Autodesk Inventor part; units mm, degrees
ref_plane "YZ Plane" through (0, 0, 0) normal (1, 0, 0) x (0, 1, 0)
ref_plane "XZ Plane" through (0, 0, 0) normal (0, 1, 0) x (-1, 0, 0)
ref_plane "XY Plane" through (0, 0, 0) normal (0, 0, 1) x (1, 0, 0)
ref_plane "Work Plane1" through (0, 0, 2) normal (0, 0, 1) x (1, 0, 0)
sketch "Sketch1" plane through (0, 0, 2) normal (0, 0, 1) x (1, 0, 0)
  circle A0 centre (-37.0712, 14) radius 3.25 construction
  circle A1 centre (-9.0712, -14) radius 3.25 construction
  line L0 (-21.8762, -24.9) -> (-21.8762, -17.08) construction
  line L1 (-21.8762, -17.08) -> (-20.0712, -17.08) construction
  arc A2 (-20.0712, -17.08) -> (-20.0712, -14.08) centre (-20.0712, -15.58) ccw construction
  line L2 (-20.0712, -14.08) -> (-21.8762, -14.08) construction
  line L3 (-21.8762, -14.08) -> (-21.8762, -3.0223) construction
  arc A3 (-21.8762, -3.0223) -> (-25.9925, 1.4242) centre (-23.0712, 0) ccw construction
  line L4 (-25.9925, 1.4242) -> (-37.0712, 1.4242) construction
  line L5 (-37.0712, 1.4242) -> (-37.0712, 3) construction
  arc A4 (-37.0712, 3) -> (-40.0712, 3) centre (-38.5712, 3) ccw construction
  line L6 (-40.0712, 3) -> (-40.0712, 1.4242) construction
  line L7 (-40.0712, 1.4242) -> (-47.9712, 1.4242) construction
  line L8 (-47.9712, 1.4242) -> (-47.9712, 17) construction
  line L9 (-47.9712, 17) -> (-44.3964, 17) construction
  line L10 (-44.3964, 17) -> (-40.0712, 21.3252) construction
  line L11 (-40.0712, 21.3252) -> (-40.0712, 24.9) construction
  line L12 (-40.0712, 24.9) -> (-6.0712, 24.9) construction
  line L13 (-6.0712, 24.9) -> (-6.0712, 21.3252) construction
  line L14 (-6.0712, 21.3252) -> (-1.746, 17) construction
  line L15 (-1.746, 17) -> (1.8288, 17) construction
  line L16 (1.8288, 17) -> (1.8288, -17) construction
  line L17 (1.8288, -17) -> (-1.746, -17) construction
  line L18 (-1.746, -17) -> (-6.1126, -21.3666) construction
  line L19 (-6.1126, -21.3666) -> (-6.1126, -24.9) construction
  line L20 (-6.1126, -24.9) -> (-21.8762, -24.9) construction
  circle A5 centre (-37.0712, -14) radius 3.25 construction
  circle A6 centre (-23.0712, 0) radius 12.45 construction
  circle A7 centre (-23.0712, 0) radius 12.7 construction
  line L21 (-37.0712, 14) -> (-9.0712, 14) construction
  line L22 (-9.0712, 14) -> (-9.0712, -14) construction
  line L23 (-9.0712, -14) -> (-37.0712, -14) construction
  line L24 (-37.0712, -14) -> (-37.0712, 14) construction
  line L25 (-4.0712, -19) -> (-4.0712, 19)
  line L26 (-4.0712, 19) -> (-42.0712, 19)
  line L27 (-42.0712, 19) -> (-42.0712, -19)
  line L28 (-42.0712, -19) -> (-4.0712, -19)
  circle A8 centre (-23.0712, 0) radius 12.8
  point P0 (0, 0)
  dimension "d0" = 5
  dimension "d1" = 0.1
extrude "Extrusion1" add sketch "Sketch1" along normal blind 6
sketch "Sketch2" plane through (0, 0, 2) normal (0, 0, -1) x (-1, 0, 0)
  circle A0 centre (23.0712, 0) radius 12.8
  circle A1 centre (23.0712, 0) radius 8.5824
  point P0 (0, 0)
extrude "Extrusion2" add sketch "Sketch2" against normal blind 0.5
sketch "Sketch3" plane through (0, 0, 2) normal (0, 0, -1) x (-1, 0, 0)
  circle A0 centre (9.0712, -14) radius 1.45 construction
  circle A1 centre (9.0712, -14) radius 2.45
  circle A2 centre (37.0712, -14) radius 1.45
  circle A3 centre (37.0712, -14) radius 1.95
  point P0 (0, 0)
  dimension "d8" = 1
  dimension "d10" = 0.5
sketch "Sketch5" plane through (0, 0, 2) normal (0, 0, -1) x (-1, 0, 0)
  arc A0 (20.0712, -14.08) -> (20.0712, -17.08) centre (20.0712, -15.58) ccw
  arc A1 (26.0712, -17.08) -> (26.0712, -14.08) centre (26.0712, -15.58) ccw
  line L0 (37.0712, 3) -> (37.0712, -3)
  arc A2 (37.0712, -3) -> (40.0712, -3) centre (38.5712, -3) ccw
  line L1 (40.0712, -3) -> (40.0712, 3)
  arc A3 (40.0712, 3) -> (37.0712, 3) centre (38.5712, 3) ccw
  line L2 (26.0712, -14.08) -> (20.0712, -14.08)
  arc A4 (20.0712, -14.08) -> (20.0712, -17.08) centre (20.0712, -15.58) ccw
  line L3 (20.0712, -17.08) -> (26.0712, -17.08)
  arc A5 (26.0712, -17.08) -> (26.0712, -14.08) centre (26.0712, -15.58) ccw
  circle A6 centre (37.0712, -14) radius 1.45
  circle A7 centre (23.0712, 0) radius 1.45
  circle A8 centre (9.0712, -14) radius 1.45
  circle A9 centre (37.0712, 14) radius 1.45
  line L4 (-1.8288, -17) -> (-1.8288, 17)
  line L5 (-1.8288, 17) -> (1.746, 17)
  line L6 (1.746, 17) -> (6.0712, 21.3252)
  line L7 (6.0712, 21.3252) -> (6.0712, 24.9)
  line L8 (6.0712, 24.9) -> (40.0712, 24.9)
  line L9 (40.0712, 24.9) -> (40.0712, 21.3252)
  line L10 (40.0712, 21.3252) -> (44.3964, 17)
  line L11 (44.3964, 17) -> (47.9712, 17)
  line L12 (47.9712, 17) -> (47.9712, -17)
  line L13 (44.3964, -17) -> (47.9712, -17)
  line L14 (40.0712, -21.3252) -> (44.3964, -17)
  line L15 (40.0712, -24.9) -> (40.0712, -21.3252)
  line L16 (6.1126, -24.9) -> (40.0712, -24.9)
  line L17 (6.1126, -24.9) -> (6.1126, -21.3666)
  line L18 (6.1126, -21.3666) -> (1.746, -17)
  line L19 (1.746, -17) -> (-1.8288, -17)
  point P0 (0, 0)
  point P1 (40.0712, -3)
extrude "Extrusion5" cut sketch "Sketch5" against normal blind 8 contours L2 A1 L3 A0 | A3 L1 A2 L0
sketch "Sketch6" plane through (-42.0712, -19, 8) normal (0, -1, 0) x (1, 0, 0)
  line L0 (0, -6) -> (38, -6)
  line L1 (38, -6) -> (38, 0)
  line L2 (0, 0) -> (38, 0)
  line L3 (0, -6) -> (0, 0)
  line L4 (31.8, 0) -> (31.8, 0)
  circle A0 centre (19, -0.9548) radius 1.45
  point P0 (42.0712, -8)
  point P1 (4.5, 0)
  dimension "d34" = 2.9
extrude "Extrusion6" cut sketch "Sketch6" against normal blind 8 contours A0 L2 | L2 A0
pattern_circular "Circular Pattern1" count 2 over 90 about axis through (-23.0712, 0, 2) along (0, 0, -1) of "Extrusion6"
chamfer "Chamfer1" distance 3 angle 45 4 edges at (-42.0712, 19, 5) (-4.0712, 19, 5) (-4.0712, -19, 5) (-42.0712, -19, 5)
hole "Hole1" at (-37.0712, -14, 2) direction (0, 0, 1) diameter 4 depth 0.1 tip angle 115
sketch "Sketch4" plane through (-4.0712, -19, 2) normal (1, 0, 0) x (0, 0, -1)
  line L0 (2, 4.45) -> (6, 4.45)
  line L1 (2, 1.55) -> (6, 1.55)
  line L2 (0, 0) -> (0, 38)
  arc A0 (2, 19) -> (2, 19) centre (1.5, 4.4206) ccw
  line L3 (-1.3741, 5) -> (-0.1, 7)
  line L4 (-1.3741, 5) -> (-0.1, 3)
  line L5 (-0.1, 7) -> (0.6045, 7)
  line L6 (0.6045, 7) -> (0.6045, 3)
  line L7 (0.6045, 3) -> (-0.1, 3)
  line L8 (-0.1, 3) -> (-0.1, 7)
extrude "Extrusion4" cut sketch "Sketch4" against normal blind 8 contours L7 L8 L5 L2 | L2 L5 L6 L7 | L4 L3 L8
properties part number "20_Cube_Insert_Kinematic_Mirrormount_90_pro_v3"
Build history of the part. All positions in model axes, mm. A direction names the side the tool comes from. Round coordinates to 2 decimals unless told otherwise and drop trailing zeros. Write each loop counter-clockwise with the first axis right and the second up, starting at its lowest first coordinate (ties: lowest second). Pieces come first, ordered by that corner, then holes. Notation, with made-up numbers: (-39, -28) -> (9, -28) arc R14 cw to (9, -22) -> close; hole circle Ø8 at (19, 27.25). An arc over 180 degrees is marked (long way). Put each result on its own line as item: value.
Item 1: Slice it at A-A, the plane z = 4. Give the cut face in (x, y).
Here are the results:
outline: (-42.07, -16) -> (-39.07, -19) -> (-7.07, -19) -> (-4.07, -16) -> (-4.07, 16) -> (-7.07, 19) -> (-39.07, 19) -> (-42.07, 16) -> close; hole (-40.07, -3) arc R1.5 ccw to (-37.07, -3) -> (-37.07, 3) arc R1.5 ccw to (-40.07, 3) -> close; hole circle Ø25.6 at (-23.07, 0); hole (-26.07, -17.08) -> (-20.07, -17.08) arc R1.5 ccw to (-20.07, -14.08) -> (-26.07, -14.08) arc R1.5 ccw to start
Item 2: Two-plate mould, pull along X, no slides. Class faces 1 (the face through (-12.071, -14, 3)), 2 (the face through (-40.071, 0, 4)), 3 (the face through (-31.4, -2.7, 2.5)), 4 (the face through (-40.59, -17.48, 4.96)): pulls with the +X half, pulls with the -X half, needs draft (parallel to the pull), parting line crosses it, or undercut.
Here are the results:
face 1: pulls with the +X half
face 2: undercut
face 3: undercut
face 4: pulls with the -X half
Item 3: Tool access for faces 5 (the face through (-37.071, 0, 4)), 6 (the face through (-11.247, 4.902, 5.212)), 7 (the face through (-36.439, 0.046, 5.596)): list every direction of +Z, -Z, +X, -X, +Y, -Y with a clear straight run to the whole face (end or side of a thin tool).
Here are the results:
face 5: +Z, -Z
face 6: +Z
face 7: -X
Item 4: Slice it at B-B, the plane x = -25. Give the cut face in (y, z).
Here are the results:
outline: (-19, 2) -> (-17.08, 2) -> (-17.08, 8) -> (-19, 8) -> close; (-14.08, 2) -> (-8.36, 2) -> (-8.36, 2.5) -> (-12.65, 2.5) -> (-12.65, 8) -> (-14.08, 8) -> close; (8.36, 2) -> (19, 2) -> (19, 8) -> (12.65, 8) -> (12.65, 2.5) -> (8.36, 2.5) -> close
Item 5: Wall check: probe 1 along X at (y, z) = (0, 4.45); probe 2 along X at (y, z) = (-1.5, 4.5); probe 3 along Y at (x, z) = (-32, 4.5). Give the ranges that are in metal, low to high. Write a range as from..to.
Here are the results:
probe 1: x = -42.07..-40.07, -37.07..-35.87, -10.27..-4.07
probe 2: x = -42.07..-40.07, -37.07..-35.78, -10.36..-4.07
probe 3: y = -19..-9.17, 9.17..19
Item 6: Flat gauge pins, fed straight in: P1, Ø13, axis at x = -25, y = -2.5, coming from the +Z side; P2, Ø1.7, axis at x = -23.07, z = 7.05, coming from the -Y side; P3, Ø0.7, axis at y = -14, z = 2.5, coming from the +X side. Where does each tip first touch, or does it go through?
Here are the results:
P1: stops at z = 2.5
P2: stops at y = 12.77
P3: stops at x = -12.07
Item 7: Slice it at C-C, the plane y = -7. Give the cut face in (x, z).
Here are the results:
outline: (-42.07, 2) -> (-28.04, 2) -> (-28.04, 2.5) -> (-33.79, 2.5) -> (-33.79, 8) -> (-42.07, 8) -> close; (-18.11, 2) -> (-4.07, 2) -> (-4.07, 8) -> (-12.35, 8) -> (-12.35, 2.5) -> (-18.11, 2.5) -> close
Item 8: Slice it at D-D, the plane y = 2. Give the cut face in (x, z), plus the area to 3 significant figures.
Here are the results:
outline: (-42.07, 2) -> (-40.07, 2) -> (-40.07, 8) -> (-42.07, 8) -> close; (-37.07, 2) -> (-31.42, 2) -> (-31.42, 2.5) -> (-35.71, 2.5) -> (-35.71, 8) -> (-37.07, 8) -> close; (-14.73, 2) -> (-4.07, 2) -> (-4.07, 8) -> (-10.43, 8) -> (-10.43, 2.5) -> (-14.73, 2.5) -> close
area: 62.6 mm^2
